from build123d import *

# Parameters (mm, degrees)
F0_W     = 41
F0_H     = 41
F0_R     = 1.5
F1_DEPTH = 4
F2_R     = 5
F3_W     = 41
F3_H     = 27.909843
F3_H_2   = 4
F4_DEPTH = 4
F5_R     = 5


with BuildPart() as f1:
    # F0 (on Top) → F1 (new body)
    with BuildSketch(Plane.XY):
        Rectangle(F0_W, F0_H)
        with Locations((-15.5, -15.5)):
            Circle(F0_R, mode=Mode.SUBTRACT)
        with Locations((15.5, -15.5)):
            Circle(F0_R, mode=Mode.SUBTRACT)
        with BuildLine():
            ThreePointArc((-14.43934, 14.43934), (-16.56066, 14.43934), (-16.56066, 16.56066))
            ThreePointArc((-16.56066, 16.56066), (-14.925975, 16.885819), (-14, 15.5))
            ThreePointArc((-14, 15.5), (-14.114181, 14.925975), (-14.43934, 14.43934))
        make_face(mode=Mode.SUBTRACT)
        with BuildLine():
            ThreePointArc((12.5, 0), (-4.783543, -11.548494), (-8.838835, 8.838835))
            ThreePointArc((-8.838835, 8.838835), (4.783543, 11.548494), (12.5, 0))
        make_face(mode=Mode.SUBTRACT)
        with Locations((15.5, 15.5)):
            Circle(F0_R, mode=Mode.SUBTRACT)
    extrude(amount=F1_DEPTH)

    # F2
    f2_edges = [f1.edges().sort_by_distance(p)[0] for p in [
        (-20.5, 20.5, 2),
        (20.5, 20.5, 2),
    ]]
    fillet(f2_edges, radius=F2_R)

    # F3 (on face) → F4 (join)
    with BuildSketch(Plane.XZ.offset(20.5)):
        with Locations((0, 17.954921)):
            Rectangle(F3_W, F3_H)
        with BuildLine():
            Line((-15.738551, 14.909843), (-15.738551, 26.909843))
            ThreePointArc((-15.738551, 26.909843), (-14.238551, 28.409843), (-12.738551, 26.909843))
            Line((-12.738551, 26.909843), (-12.738551, 14.909843))
            ThreePointArc((-12.738551, 14.909843), (-14.238551, 13.409843), (-15.738551, 14.909843))
        make_face(mode=Mode.SUBTRACT)
        with BuildLine():
            ThreePointArc((12.738551, 26.909843), (14.238551, 28.409843), (15.738551, 26.909843))
            Line((15.738551, 26.909843), (15.738551, 14.909843))
            ThreePointArc((15.738551, 14.909843), (14.238551, 13.409843), (12.738551, 14.909843))
            Line((12.738551, 14.909843), (12.738551, 26.909843))
        make_face(mode=Mode.SUBTRACT)
        with Locations((0, 2)):
            Rectangle(F3_W, F3_H_2)
    extrude(amount=F4_DEPTH)

    # F5
    f5_edges = [f1.edges().sort_by_distance(p)[0] for p in [
        (20.5, -22.5, 31.909843),
        (-20.5, -22.5, 31.909843),
    ]]
    fillet(f5_edges, radius=F5_R)


solid = f1.part
Check sheet for the modelled part. Datum: model origin and axes. Units: mm. A direction names the side the tool comes from. Give positions to 0.01 mm unless a question says otherwise; leave off trailing zeros. Loops run counter-clockwise (first coordinate to the right, second up) from the corner with the lowest first, then second, coordinate; pieces in that order, holes last. Notation, with made-up numbers: M 20,14 L 66,14 A24 ccw 66,40 Z; hole C -32.75,62 d9. An arc over 180 degrees is marked long. Answer as a JSON object with one key per item and string values. Group by question number.
Q1. Access from +Z, -Z, +X, -X, +Y, -Y to the whole of each face (thin tool, end or side, straight path). Record for faces 5 (the cylindrical face through (-14.27, -22.47, 28.41)), 6 (the flat face through (-9, 9, 4)), 7 (the flat face through (-20.5, -11.8, 3.6)).
Q2. Go/stop test with flat-tipped pins: P1, Ø6, axis at x = -10, y = -12.5, coming from the +Z side; P2, Ø4, axis at x = 11.5, z = 25.5, coming from the +Y side; P3, Ø2.5, axis at x = 15.5, y = -15.5, coming from the +Z side; P4, Ø6, axis at y = -18.5, z = 21, coming from the +X side. Record where each tip stops, or that it passes through.
Q3. Cross-section at D-D on x = 9.5. Record the cut outline in (y, z).
Q4. Cross-section at B-B on y = 11. Record the cut outline in (x, z), then the cut area to 3 significant figures.
Q5. Cross-section at A-A on x = -7.5. Record the cut outline in (y, z).
Q6. Release check for a two-part mould opening along X. For faces 1 (the cylindrical face through (-17, -15.43, 1.97)), 2 (the cylindrical face through (-19.07, 19, 2.03)), 3 (the cylindrical face through (19, -22.53, 30.48)), 4 (the flat face through (0, -20.5, 18)) record: released by +X, released by -X, zero draft, split by the parting line, or undercut.
Q7. Material ranges on line 1 along Y through (x, z) = (15.5, 3.15); line 2 along Y through (x, z) = (0, 2.5); line 3 along Z through (x, y) = (8, -11), recorded low to high. Write a range as [from, to].
Q8. Cross-section at C-C on z = 27.5. Record the cut outline in (x, y), then the cut area to 3 significant figures.
Evaluation:
{
 "1": {"face 5": "+Y, -Y", "face 6": "+Z, +X, -X, +Y", "face 7": "+Z, -Z, -X, +Y, -Y"},
 "2": {"P1": "stops at z = 4", "P2": "stops at y = -20.5", "P3": "passes through", "P4": "stops at x = 20.5"},
 "3": {"outline": "M -24.5,0 L -8.12,0 L -8.12,4 L -20.5,4 L -20.5,31.91 L -24.5,31.91 Z; M 8.12,0 L 20.5,0 L 20.5,4 L 8.12,4 Z"},
 "4": {"outline": "M -20.5,0 L -5.94,0 L -5.94,4 L -20.5,4 Z; M 5.94,0 L 20.5,0 L 20.5,4 L 5.94,4 Z", "area": "117 mm2"},
 "5": {"outline": "M -24.5,0 L -10,0 L -10,4 L -20.5,4 L -20.5,31.91 L -24.5,31.91 Z; M 10,0 L 20.5,0 L 20.5,4 L 10,4 Z"},
 "6": {"face 1": "undercut", "face 2": "released by -X", "face 3": "released by +X", "face 4": "zero draft"},
 "7": {"line 1": "y = [-24.5, -17], [-14, 14], [17, 20.5]", "line 2": "y = [-24.5, -12.5], [12.5, 20.5]", "line 3": "z = [0, 4]"},
 "8": {"outline": "M -20.47,-24.5 L -15.62,-24.5 L -15.62,-20.5 L -20.47,-20.5 Z; M -12.86,-24.5 L 12.86,-24.5 L 12.86,-20.5 L -12.86,-20.5 Z; M 15.62,-24.5 L 20.47,-24.5 L 20.47,-20.5 L 15.62,-20.5 Z", "area": "142 mm2"}
}
